```python
from build123d import *

# Parameters (mm, degrees)
SKETCH1_R               = 7.5
BOSS_EXTRUDE1_DEPTH     = 15
SKETCH2_R               = 7.5
BOSS_EXTRUDE2_DEPTH     = 50
SKETCH3_W               = 50
SKETCH3_H               = 40
BOSS_EXTRUDE3_DEPTH     = 65
CUT_EXTRUDE1_DEPTH      = 105.024035684
CUT_EXTRUDE2_DEPTH      = 96.372952141
SKETCH9_R               = 4
CUT_EXTRUDE3_DEPTH      = 104.107953137
CUT_EXTRUDE4_DEPTH      = 95.272212237
CUT_EXTRUDE4_DEPTH_BACK = 95.272212237
SKETCH10_R              = 1.6


with BuildPart() as part:
    # Sketch1 → Boss-Extrude1 (new body)
    with BuildSketch(Plane.XY):
        with BuildLine():
            Line((0, 0), (50, 0))
            Line((50, 0), (50, 50))
            ThreePointArc((50, 50), (40.582575695, 63.228756555), (25, 58.660254038))
            ThreePointArc((25, 58.660254038), (9.417424305, 63.228756555), (0, 50))
            Line((0, 50), (0, 0))
        make_face()
        with Locations((36, 50)):
            Circle(SKETCH1_R, mode=Mode.SUBTRACT)
        with Locations((14, 50)):
            Circle(SKETCH1_R, mode=Mode.SUBTRACT)
    extrude(amount=BOSS_EXTRUDE1_DEPTH)

    # Sketch2 → Boss-Extrude2 (add)
    with BuildSketch(Plane.XY.offset(15)):
        with BuildLine():
            Line((25, 50), (25, 0))
            Line((25, 0), (50, 0))
            Line((50, 0), (50, 50))
            ThreePointArc((50, 50), (37.5, 62.5), (25, 50))
        make_face()
        with Locations((36, 50)):
            Circle(SKETCH2_R, mode=Mode.SUBTRACT)
    extrude(amount=BOSS_EXTRUDE2_DEPTH)

    # Sketch3 → Boss-Extrude3 (add)
    with BuildSketch(Plane(origin=(0, 0, 0), x_dir=(-1, 0, 0), z_dir=(0, 0, -1))):
        with Locations((-25, 20)):
            Rectangle(SKETCH3_W, SKETCH3_H)
    extrude(amount=-BOSS_EXTRUDE3_DEPTH)

    # Sketch4 → Cut-Extrude1 (cut, through all)
    with BuildSketch(Plane.ZY):
        with BuildLine():
            Line((23, 36), (43, 36))
            ThreePointArc((43, 36), (53, 26), (43, 16))
            Line((43, 16), (23, 16))
            ThreePointArc((23, 16), (13, 26), (23, 36))
        make_face()
    extrude(amount=-CUT_EXTRUDE1_DEPTH, mode=Mode.SUBTRACT)

    # Sketch2_3 → Cut-Extrude2 (cut, through all)
    with BuildSketch(Plane.XY.offset(15)):
        with BuildLine():
            ThreePointArc((50, 50), (37.5, 62.5), (25, 50))
            ThreePointArc((25, 50), (12.5, 62.5), (0, 50))
            ThreePointArc((0, 50), (9.417424305, 63.228756555), (25, 58.660254038))
            ThreePointArc((25, 58.660254038), (40.582575695, 63.228756555), (50, 50))
        make_face()
    extrude(amount=-CUT_EXTRUDE2_DEPTH, mode=Mode.SUBTRACT)

    # Sketch9 → Cut-Extrude3 (cut, through all)
    with BuildSketch(Plane.ZY):
        with Locations((7, 13)):
            Circle(SKETCH9_R)
        with Locations((58, 13)):
            Circle(SKETCH9_R)
    extrude(amount=-CUT_EXTRUDE3_DEPTH, mode=Mode.SUBTRACT)

    # Sketch10 → Cut-Extrude4 (cut, two sides: drawn at the far end of the back side and taken through both)
    with BuildSketch(Plane(origin=(0, 16, 0), x_dir=(1, 0, 0), z_dir=(0, 1, 0)).offset(-CUT_EXTRUDE4_DEPTH_BACK)):
        with Locations(Location((9.306144925, -33, 0), (0, 0, 90))):
            Circle(SKETCH10_R)
    extrude(amount=CUT_EXTRUDE4_DEPTH + CUT_EXTRUDE4_DEPTH_BACK, mode=Mode.SUBTRACT)


solid = part.part
```
Source: CAD feature listing. Evaluate the final solid. Frame: model axes, mm. A direction names the side the tool comes from. Coordinates: 2 decimals unless noted, no trailing zeros. Write each loop counter-clockwise with the first axis right and the second up, starting at its lowest first coordinate (ties: lowest second). Pieces come first, ordered by that corner, then holes. Notation, with made-up numbers: (89, 10) -> (96, 10) arc R20 ccw to (96, 18) -> close; hole circle Ø11 at (-25.5, 50.5). An arc over 180 degrees is marked (long way). Return JSON: item names as keys, results as strings. Group by question number.
1) Contact query for flat-ended pins moving along their axis: P1, Ø1.5, axis at y = 44.5, z = 46, coming from the -X side; P2, Ø12.5, axis at x = 13, z = 36.5, coming from the +Y side; P3, Ø1, axis at y = 55, z = 25.5, coming from the +X side. Output: stop coordinate, or through.
2) Section query C-C, the plane z = 7. Return loops of the section in (x, y).
3) Section query B-B, the plane y = 26. Return loops of the section in (x, z), plus the area to 3 significant figures.
4) Set-up query: faces 1 (the face through (25, 16, 33)), 2 (the face through (0, 14, 32)), 3 (the face through (7, 54, 15)). Return all of +Z, -Z, +X, -X, +Y, -Y with unobstructed straight access to the full face (end or side cutting, diameter ignored); none if empty.
5) Mould query, pull axis Y, two halves, no side actions, for faces 4 (the face through (25, 45, 40)), 5 (the face through (25, 0, 32)), 6 (the face through (24.65, 14.201, 61.815)), 7 (the face through (25, 26, 13)). Classes: +Y half, -Y half, draft (parallel to the pull), parting line (faces both ways), or undercut.
6) Section query A-A, the plane z = 27. Return loops of the section in (x, y), plus the area to 3 significant figures.
7) Section query D-D, the plane x = 36. Return loops of the section in (y, z).
8) Ray query, line 1 along Y through (x, z) = (41, 23.5); line 2 along Y through (x, z) = (30.5, 54.5); line 3 along Z through (x, y) = (38.5, 14.5). Return the intervals inside material, ascending.
From the geometry:
{
 "1": {"P1": "x = 25", "P2": "y = 40", "P3": "x = 49.16"},
 "2": {"outline": "(0, 0) -> (50, 0) -> (50, 9) -> (0, 9) -> close; (0, 17) -> (50, 17) -> (50, 50) arc R12.5 ccw to (25, 50) arc R12.5 ccw to (0, 50) -> close; hole circle Ø15 at (14, 50); hole circle Ø15 at (36, 50)"},
 "3": {"outline": "(0, 0) -> (50, 0) -> (50, 13) -> (0, 13) -> close; (0, 53) -> (50, 53) -> (50, 65) -> (0, 65) -> close", "area": "1,250 mm²"},
 "4": {"face 1": "+X, -X", "face 2": "+Z, -Z, -X, +Y, -Y", "face 3": "+Z, -X, +Y"},
 "5": {"face 4": "draft", "face 5": "-Y half", "face 6": "undercut", "face 7": "undercut"},
 "6": {"outline": "(0, 0) -> (50, 0) -> (50, 16) -> (0, 16) -> close; (0, 36) -> (50, 36) -> (50, 50) arc R12.5 ccw to (25, 50) -> (25, 40) -> (0, 40) -> close; hole circle Ø15 at (36, 50)", "area": "1,320 mm²"},
 "7": {"outline": "(0, 0) -> (42.5, 0) -> (42.5, 65) -> (0, 65) -> close; (57.5, 0) -> (62.41, 0) -> (62.41, 65) -> (57.5, 65) -> close; hole circle Ø8 at (13, 7); hole circle Ø8 at (13, 58); hole (16, 23) arc R10 ccw to (36, 23) -> (36, 43) arc R10 ccw to (16, 43) -> close"},
 "8": {"line 1": "0 to 16, 36 to 44.41, 55.59 to 62", "line 2": "0 to 11.06, 14.94 to 44.9, 55.1 to 60.36", "line 3": "0 to 3.29, 10.71 to 54.29, 61.71 to 65"}
}
